from build123d import *

# Parameters (mm, degrees)
BOSS_EXTRUDE1_DEPTH = 139.7
SKETCH3_R           = 6.35
BOSS_EXTRUDE2_DEPTH = 6.35
FILLET1_R           = 6.35
CHAMFER1_SIZE       = 2.54
SKETCH4_W           = 9.672441956
SKETCH4_H           = 22.08614384
CUT_EXTRUDE1_DEPTH  = 152.4


# Some blends are built 0.0001 mm under size
with BuildPart() as part:
    # Sketch1 → Boss-Extrude1 (new body)
    with BuildSketch(Plane(origin=(0, 0, 0), x_dir=(1, 0, 0), z_dir=(0, 1, 0))):
        Polygon((0, 3.666174209), (-3.175, 1.833087105), (-3.175, -1.833087105), (0, -3.666174209), (3.175, -1.833087105), (3.175, 1.833087105), align=None)
    extrude(amount=BOSS_EXTRUDE1_DEPTH)

    # Sketch3 → Boss-Extrude2 (add)
    with BuildSketch(Plane(origin=(0, 139.7, 0), x_dir=(1, 0, 0), z_dir=(0, 1, 0))):
        with Locations(Location((0, 0, 0), (0, 0, 270))):
            Circle(SKETCH3_R)
    extrude(amount=BOSS_EXTRUDE2_DEPTH)

    # Fillet1
    fillet1_edges = [part.edges().sort_by_distance(p)[0] for p in [
        (0, 146.05, -6.35),
    ]]
    fillet(fillet1_edges, radius=FILLET1_R - 0.0001)  # a hair under: the kernel refuses the full size

    # Chamfer1
    # the kernel refuses this chamfer: 2.54 mm, written as the material it takes off along each edge
    with BuildSketch(Plane(origin=(0, 139.7, 0), x_dir=(0, 0, 1), z_dir=(-1, 0, 0))) as chamfer1_piece_1:
        Polygon((6.35, CHAMFER1_SIZE), (6.35 - CHAMFER1_SIZE, 0), (6.35, 0), align=None)
    revolve(axis=Axis((0, 139.7, 0), (0, 1, 0)), mode=Mode.SUBTRACT)

    # Sketch4 → Cut-Extrude1 (cut)
    with BuildSketch(Plane.XZ):
        with Locations((-8.011220978, 1.321657353)):
            Rectangle(SKETCH4_W, SKETCH4_H)
    extrude(amount=-CUT_EXTRUDE1_DEPTH, mode=Mode.SUBTRACT)


solid = part.part
Check sheet for the modelled part. Datum: model origin and axes. Units: mm. A direction names the side the tool comes from. Round coordinates to 2 decimals unless told otherwise and drop trailing zeros. Loops run counter-clockwise (first coordinate to the right, second up) from the corner with the lowest first, then second, coordinate; pieces in that order, holes last. Notation, with made-up numbers: M 2,-16.5 L 35,-16.5 A27 cw 35,22.5 Z; hole C -39,32.5 d2. An arc over 180 degrees is marked long. One line per question, with ' | ' between items. Start each with the question number.
Item 1: Section check A-A (y = 47). Record the boundary of the cut face in (x, z) (3 decimals).
Item 2: Scan lines: probe 1 along Y at (x, z) = (-1, 3); probe 2 along X at (y, z) = (134, 1) (3 decimals); probe 3 along Z at (x, y) = (1.5, 17). Record each from-to range of solid material in increasing order.
Item 3: Set-up check for faces 1 (the face through (-1.57, 68.87, -2.76)), 2 (the face through (-1.61, 68.872, 2.737)), 3 (the face through (3.175, 69, 0)): record each of +Z, -Z, +X, -X, +Y, -Y from which the full face is reachable in a straight line by a thin tool's end or side.
Item 4: Gauge pin test, flat ends, axial feed: pin 1 Ø2 at (x, z) = (1.5, 0) entering from -Y; pin 2 Ø1 at (x, y) = (2.5, 107.5) entering from -Z; pin 3 Ø2 at (y, z) = (108.5, 4.5) entering from +X; pin 4 Ø2 at (x, z) = (3.5, 4) entering from +Y. Record the tip position at first contact, or that the pin passes through.
Worked out:
1) outline: M -3.175,-1.833 L 0,-3.666 L 3.175,-1.833 L 3.175,1.833 L 0,3.666 L -3.175,1.833 Z
2) probe 1: 0 to 145.21 | probe 2: -3.175 to 3.175 | probe 3: -2.8 to 2.8
3) face 1: -Z, -X, -Y | face 2: +Z, -X, -Y | face 3: +Z, -Z, +X, -Y
4) pin 1: y = 0 | pin 2: z = -2.51 | pin 3: x = 0.29 | pin 4: y = 144.36
